from build123d import *

# Parameters (mm, degrees)
SKETCH1_R           = 1.5
BOSS_EXTRUDE3_DEPTH = 3.85


with BuildPart() as part:
    # Sketch1 → Boss-Extrude3 (new body, symmetric)
    with BuildSketch(Plane(origin=(0, 0, 0), x_dir=(1, 0, 0), z_dir=(0, 1, 0))):
        with BuildLine():
            Line((-13.75, -5.4), (0, -5.4))
            Line((0, -5.4), (0, 0))
            ThreePointArc((0, 0), (-3.769352362, 10.315583277), (0, 20.631166554))
            Line((0, 20.631166554), (0, 28.431166554))
            Line((0, 28.431166554), (-1, 28.431166554))
            ThreePointArc((-1, 28.431166554), (-2.610090465, 27.962492036), (-3.717108681, 26.702905684))
            Line((-3.717108681, 26.702905684), (-13.467108681, 5.87173913))
            ThreePointArc((-13.467108681, 5.87173913), (-13.6784233, 5.251411528), (-13.75, 4.6))
            Line((-13.75, 4.6), (-13.75, -5.4))
        make_face()
        with Locations((-10.75, -2.4)):
            Circle(SKETCH1_R, mode=Mode.SUBTRACT)
        with Locations((-3, -2.4)):
            Circle(SKETCH1_R, mode=Mode.SUBTRACT)
    extrude(amount=BOSS_EXTRUDE3_DEPTH, both=True)


solid = part.part
CAD build for the part. Positions are in the model's coordinates, mm. Round coordinates to 2 decimals unless told otherwise and drop trailing zeros. Write each loop counter-clockwise with the first axis right and the second up, starting at its lowest first coordinate (ties: lowest second). Pieces come first, ordered by that corner, then holes. Notation, with made-up numbers: M -13.5,-39 L 28.5,-39 A29 ccw 28.5,-14 Z; hole C -16,-38 d10. An arc over 180 degrees is marked long. Use a Markdown table: item, result. Add a question column.
1. Slice it at D-D on x = -10.75. Give the cut face in (y, z).
2. Slice it at C-C on x = -2.75. Give the cut face in (y, z).
3. Slice it at A-A on z = 2.4. Give the cut face in (x, y), then the cut area to 3 significant figures.
4. Pull direction X, two halves, no side cores. Call faces 1 (the face through (0, 0, -24)), 2 (the face through (-7, -3.85, -8)), 3 (the face through (-1.57, -0.05, 1.95)): released by +X, released by -X, zero draft, split by the parting line, or undercut.
5. Drill centre lines: probe 1 along X at (y, z) = (1.25, 2.4); probe 2 along Z at (x, y) = (-4, -3); probe 3 along Z at (x, y) = (-2.5, 2.75). Where is each one in solid material? Low to high.
6. Slice it at B-B on y = 0.75. Give the cut face in (x, z).
7. Flat gauge pin, fed straight in: P1, Ø1.5, axis at x = -8, y = 0.5, coming from the -Z side. Where does the tip first touch, or does it go through?
Reply:
| question | item | result |
|---|---|---|
| 1 | outline | M -3.85,-11.68 L 3.85,-11.68 L 3.85,0.9 L -3.85,0.9 Z; M -3.85,3.9 L 3.85,3.9 L 3.85,5.4 L -3.85,5.4 Z |
| 2 | outline | M -3.85,-27.87 L 3.85,-27.87 L 3.85,-15.94 L -3.85,-15.94 Z; M -3.85,-4.7 L 3.85,-4.7 L 3.85,0.92 L -3.85,0.92 Z; M -3.85,3.88 L 3.85,3.88 L 3.85,5.4 L -3.85,5.4 Z |
| 3 | outline | M -13.75,-3.85 L -12.25,-3.85 L -12.25,3.85 L -13.75,3.85 Z; M -9.25,-3.85 L -4.5,-3.85 L -4.5,3.85 L -9.25,3.85 Z; M -1.5,-3.85 L 0,-3.85 L 0,3.85 L -1.5,3.85 Z |
| 3 | area | 59.7 mm^2 |
| 4 | face 1 | released by +X |
| 4 | face 2 | zero draft |
| 4 | face 3 | undercut |
| 5 | probe 1 | x = -13.75 to -12.25, -9.25 to -4.5, -1.5 to 0 |
| 5 | probe 2 | z = -26.1 to 1.28, 3.52 to 5.4 |
| 5 | probe 3 | z = -28.03 to -16.56, -4.07 to 0.99, 3.81 to 5.4 |
| 6 | outline | M -13.75,-4.6 A3 ccw -13.47,-5.87 L -3.72,-26.7 A3 ccw -1,-28.43 L 0,-28.43 L 0,-20.63 A16 cw 0,0 L 0,5.4 L -13.75,5.4 Z; hole C -10.75,2.4 d3; hole C -3,2.4 d3 |
| 7 | P1 | stops at z = -19.15 |
